Source: CAD feature listing. Evaluate the final solid. Frame: model axes, mm. A direction names the side the tool comes from. Round coordinates to 2 decimals unless told otherwise and drop trailing zeros. Order: outer loops, then holes, each group sorted by start corner. A loop starts at its lowest first (then second) coordinate and runs counter-clockwise, first axis right, second up. Notation, with made-up numbers: (3.5, 13) -> (51.5, 13) arc R26 ccw to (51.5, 51) -> close; hole circle Ø11 at (84.25, 49). An arc over 180 degrees is marked (long way). One line per item, written item: value. Start each with the question number.
1) Section C-C (z = 30). Return the cut outline in (x, y), and give its area (3 significant figures).
2) Pin query (flat end, axial travel): P1, Ø1.2, axis at x = 0.5, z = 47, coming from the +Y side (3 decimals); P2, Ø6.5, axis at y = 0, z = 48.625, coming from the +X side; P3, Ø2.5, axis at y = -1, z = 49, coming from the -X side; P4, Ø2, axis at x = -2.5, y = 3, coming from the +Z side. Return the tip coordinate at first contact, or that it passes through.
3) Section A-A (y = 0). Return the cut outline in (x, z) (3 decimals).
4) Reachability of faces 1 (the face through (-3, -6, 42)), 2 (the face through (0, 0, 35)), 3 (the face through (0, 4.375, 46)), 4 (the face through (-2, -1.9, 46.6)) from +Z, -Z, +X, -X, +Y, -Y: full face, straight path, thin tool, end or side. Return the list, or none.
5) Mould query, pull axis Y, two halves, no side actions, for faces 5 (the face through (0, -4.375, 46)), 6 (the face through (2, -1.9, 46.6)), 7 (the face through (-0.028, -0.958, 50.934)). Classes: pulls with the +Y half, pulls with the -Y half, needs draft (parallel to the pull), parting line crosses it, or undercut.
6) Ray query, L1, parallel to Y at x = 0, z = 15; L2, parallel to X at y = -0.5, z = 16. Return the intervals inside material, ascending.
7) Section B-B (x = 0). Return the cut outline in (y, z) (3 decimals), and give its area (3 significant figures).
```python
from build123d import *

# Parameters (mm, degrees)
SKETCH2_R            = 6.6
EXTERNAL_SHOCK_DEPTH = 34
SHOCK_CHAMFER_SIZE   = 2
SKETCH3_R            = 7.85
CYLINDER_A_DEPTH     = 8
SKETCH4_R            = 6.4
CYLINDER_B_DEPTH     = 2
MOUNTING_BOSS_DEPTH  = 2
SKETCH6_R            = 2.5
MOUNTING_HOLE_DEPTH  = 4
SKETCH7_R            = 1.5
INNER_HOLE_DEPTH     = 35


with BuildPart() as part:
    # Sketch2 → External Shock (new body)
    with BuildSketch(Plane.XY):
        Circle(SKETCH2_R)
    extrude(amount=EXTERNAL_SHOCK_DEPTH)

    # Shock Chamfer
    shock_chamfer_edges = [part.edges().sort_by_distance(p)[0] for p in [
        (-6.6, 0, 0),
    ]]
    chamfer(shock_chamfer_edges, length=SHOCK_CHAMFER_SIZE)

    # Sketch3 → Cylinder A (add)
    with BuildSketch(Plane.XY.offset(34)):
        Circle(SKETCH3_R)
    extrude(amount=CYLINDER_A_DEPTH)

    # Sketch4 → Cylinder B (add)
    with BuildSketch(Plane.XY.offset(42)):
        Circle(SKETCH4_R)
    extrude(amount=CYLINDER_B_DEPTH)

    # Sketch5 → Mounting Boss (add, symmetric)
    with BuildSketch(Plane(origin=(0, 0, 0), x_dir=(0, 0, -1), z_dir=(1, 0, 0))):
        with BuildLine():
            Line((-48.625, -4.375), (-44, -4.375))
            Line((-44, -4.375), (-44, 4.375))
            Line((-44, 4.375), (-48.625, 4.375))
            ThreePointArc((-48.625, 4.375), (-53, 0), (-48.625, -4.375))
        make_face()
    extrude(amount=MOUNTING_BOSS_DEPTH, both=True)

    # Sketch6 → Mounting Hole (cut)
    with BuildSketch(Plane.ZY.offset(2)):
        with Locations((48.625, 0)):
            Circle(SKETCH6_R)
    extrude(amount=-MOUNTING_HOLE_DEPTH, mode=Mode.SUBTRACT)

    # Sketch7 → Inner Hole (cut)
    with BuildSketch(Plane(origin=(0, 0, 0), x_dir=(-1, 0, 0), z_dir=(0, 0, -1))):
        Circle(SKETCH7_R)
    extrude(amount=-INNER_HOLE_DEPTH, mode=Mode.SUBTRACT)


solid = part.part
```
Findings:
1. outline: circle Ø13.2 at (0, 0); hole circle Ø3 at (0, 0)
1. area: 130 mm2
2. P1: y = 4.375
2. P2: x = 2
2. P3: through
2. P4: z = 52.44
3. outline: (-7.85, 34) -> (-6.6, 34) -> (-6.6, 2) -> (-4.6, 0) -> (-1.5, 0) -> (-1.5, 35) -> (1.5, 35) -> (1.5, 0) -> (4.6, 0) -> (6.6, 2) -> (6.6, 34) -> (7.85, 34) -> (7.85, 42) -> (6.4, 42) -> (6.4, 44) -> (2, 44) -> (2, 46.125) -> (-2, 46.125) -> (-2, 44) -> (-6.4, 44) -> (-6.4, 42) -> (-7.85, 42) -> close; (-2, 51.125) -> (2, 51.125) -> (2, 53) -> (-2, 53) -> close
4. face 1: +Z
4. face 2: -Z
4. face 3: +Z, +X, -X, +Y
4. face 4: +Z, -X, +Y, -Y
5. face 5: pulls with the -Y half
5. face 6: needs draft
5. face 7: undercut
6. L1: -6.6 to -1.5, 1.5 to 6.6
6. L2: -6.58 to -1.41, 1.41 to 6.58
7. outline: (-7.85, 34) -> (-6.6, 34) -> (-6.6, 2) -> (-4.6, 0) -> (-1.5, 0) -> (-1.5, 35) -> (1.5, 35) -> (1.5, 0) -> (4.6, 0) -> (6.6, 2) -> (6.6, 34) -> (7.85, 34) -> (7.85, 42) -> (6.4, 42) -> (6.4, 44) -> (4.375, 44) -> (4.375, 48.625) arc R4.375 ccw to (-4.375, 48.625) -> (-4.375, 44) -> (-6.4, 44) -> (-6.4, 42) -> (-7.85, 42) -> close; hole circle Ø5 at (0, 48.625)
7. area: 542 mm2
